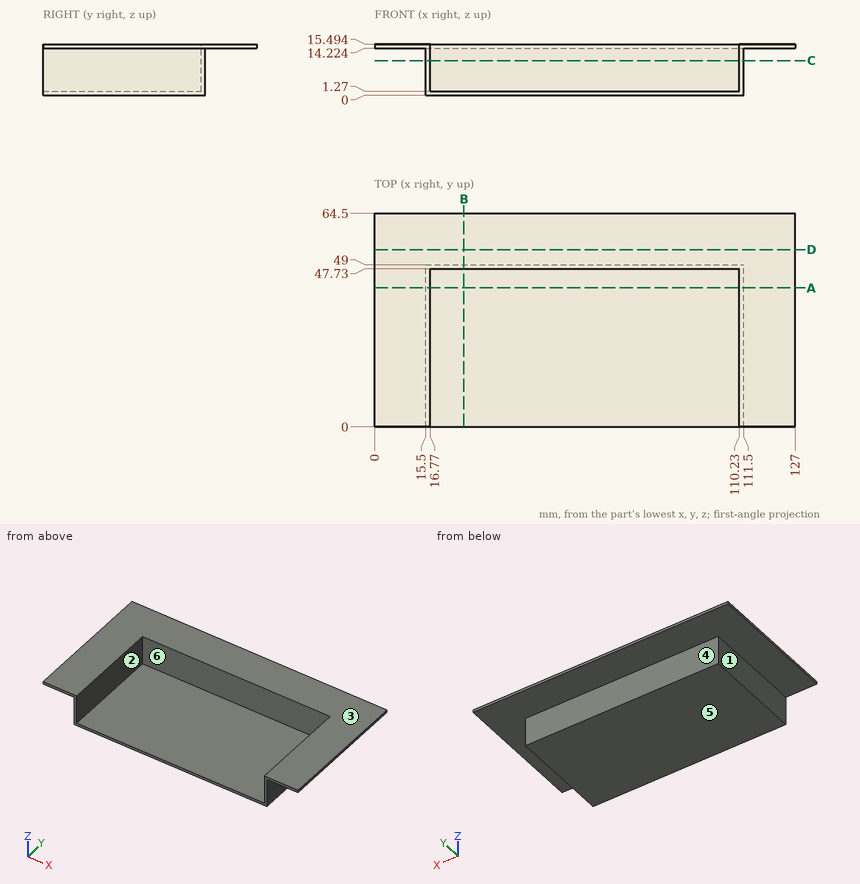
Drawing for the job (mm, zero at the part's lowest x, y, z). A direction names the side the tool comes from. Coordinates: 2 decimals unless noted, no trailing zeros. Order: outer loops, then holes, each group sorted by start corner. A loop starts at its lowest first (then second) coordinate and runs counter-clockwise, first axis right, second up. Notation, with made-up numbers: (10.25, 26) - (14.25, 26) arc R19 ccw to (14.25, 36) - close; hole circle Ø10 at (78.25, 64). An arc over 180 degrees is marked (long way). Use a Markdown table: item, result. Add a question column.
(1) Saw through at A-A (y = 42). Give the cut face in (x, z), then the cut area to 3 significant figures.
(2) Saw through at B-B (x = 27). Give the cut face in (y, z).
(3) Flat gauge pins, fed straight in: pin 1 (8 mm diameter, centred on x = 35.5, z = 5.5, fed in from -Y); pin 2 (1.5 mm diameter, centred on y = 25.5, z = 11, fed in from +X); pin 3 (4.5 mm diameter, centred on y = 33, z = 9, fed in from -X). Where does each tip first touch, or does it go through?
(4) Saw through at C-C (z = 10.5). Give the cut face in (x, y), then the cut area to 3 significant figures.
(5) Which spindle directions (+Z, -Z, +X, -X, +Y, -Y) get a long thin tool onto all of the face, cutting with end or side? Do the marked faces 4, 5 and 6. Say none if no direction does.
(6) Pull direction X, two halves, no side cores. Call the marked faces 1, 2 and 3: +X half, -X half, draft (parallel to the pull), parting line (faces both ways), or undercut.
(7) Drill centre lines: line 1 along X through (y, z) = (8, 11.75); line 2 along Y through (x, z) = (103, 0.5); line 3 along Z through (x, y) = (40, 61). Where is each one in solid material? Low to high. Write a range as [from, to].
(8) Saw through at D-D (y = 53.5). Give the cut face in (x, z), then the cut area to 3 significant figures.
Solved:
| question | item | result |
|---|---|---|
| 1 | outline | (0, 14.22) - (15.5, 14.22) - (15.5, 0) - (111.5, 0) - (111.5, 14.22) - (127, 14.22) - (127, 15.49) - (110.23, 15.49) - (110.23, 1.27) - (16.77, 1.27) - (16.77, 15.49) - (0, 15.49) - close |
| 1 | area | 197 mm² |
| 2 | outline | (0, 0) - (49, 0) - (49, 14.22) - (64.5, 14.22) - (64.5, 15.49) - (47.73, 15.49) - (47.73, 1.27) - (0, 1.27) - close |
| 3 | pin 1 | stops at y = 47.73 |
| 3 | pin 2 | stops at x = 111.5 |
| 3 | pin 3 | stops at x = 15.5 |
| 4 | outline | (15.5, 0) - (16.77, 0) - (16.77, 47.73) - (110.23, 47.73) - (110.23, 0) - (111.5, 0) - (111.5, 49) - (15.5, 49) - close |
| 4 | area | 243 mm² |
| 5 | face 4 | -Z, +X, -X, +Y |
| 5 | face 5 | -Z, +X, -X, +Y, -Y |
| 5 | face 6 | +Z, -Y |
| 6 | face 1 | -X half |
| 6 | face 2 | undercut |
| 6 | face 3 | draft |
| 7 | line 1 | x = [15.5, 16.77], [110.23, 111.5] |
| 7 | line 2 | y = [0, 49] |
| 7 | line 3 | z = [14.22, 15.49] |
| 8 | outline | (0, 14.22) - (127, 14.22) - (127, 15.49) - (0, 15.49) - close |
| 8 | area | 161 mm² |
